For this review, use the dimensioned drawing (mm, ordinates from the lowest corner) and the shaded views. A direction names the side the tool comes from. Coordinates: 2 decimals unless noted, no trailing zeros. Write each loop counter-clockwise with the first axis right and the second up, starting at its lowest first coordinate (ties: lowest second). Pieces come first, ordered by that corner, then holes. Notation, with made-up numbers: (77, 79) -> (125, 79) arc R29 cw to (125, 102) -> close; hole circle Ø7 at (31, -16). An arc over 180 degrees is marked (long way). Put each result on its own line as item: value. Start each with the question number.
Item 1: Consider section D-D on x = 11. Give the boundary of the cut face in (y, z), and give its area (3 significant figures).
Item 2: Consider section A-A on z = 16.5. Give the boundary of the cut face in (x, y).
Item 3: Consider section C-C on x = 3. Give the boundary of the cut face in (y, z), and give its area (3 significant figures).
Item 4: Consider section B-B on y = 2.5. Give the boundary of the cut face in (x, z).
Item 5: For the marked faces 1 and 2, list the 3-axis set-ups (+Z, -Z, +X, -X, +Y, -Y) from which the entire face can be reached by the end or side of a thin tool; tool diameter is ignored.
Item 6: Insertion check: P1, Ø3, axis at x = 21, z = 27.5, coming from the -Y side; P2, Ø9, axis at x = 17.5, z = 25.5, coming from the -Y side; P3, Ø12.5, axis at x = 29, y = 22.5, coming from the +Z side. Each pin has a flat end and moves straight along its axis. Give the tip position at first contact, or say it passes through.
Item 7: To check wall thickness, follow L1, parallel to Y at x = 37, z = 7; L2, parallel to Z at x = 20, y = 30.6; L3, parallel to X at y = 2, z = 3. State the ranges of each line that lie inside material, in increasing order.
Item 8: The part is to be moulded in two halves that separate along Y. For the marked faces 3, 4, 5 and 6, say which applies: +Y half, -Y half, draft (parallel to the pull), parting line (faces both ways), or undercut.
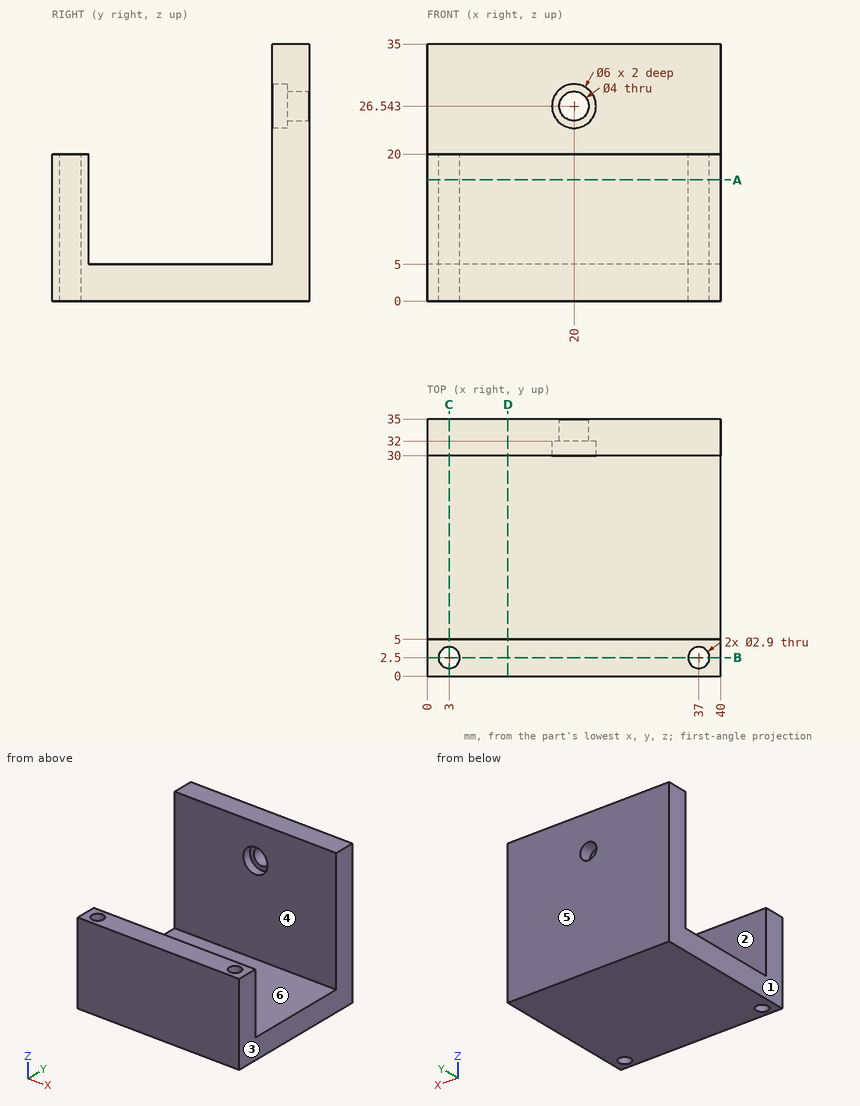
Return value:
1. outline: (0, 0) -> (35, 0) -> (35, 35) -> (30, 35) -> (30, 5) -> (5, 5) -> (5, 20) -> (0, 20) -> close
1. area: 400 mm^2
2. outline: (0, 0) -> (40, 0) -> (40, 5) -> (0, 5) -> close; (0, 30) -> (40, 30) -> (40, 35) -> (0, 35) -> close; hole circle Ø2.9 at (3, 2.5); hole circle Ø2.9 at (37, 2.5)
3. outline: (0, 0) -> (1.05, 0) -> (1.05, 20) -> (0, 20) -> close; (3.95, 0) -> (35, 0) -> (35, 35) -> (30, 35) -> (30, 5) -> (5, 5) -> (5, 20) -> (3.95, 20) -> close
3. area: 342 mm^2
4. outline: (0, 0) -> (1.55, 0) -> (1.55, 20) -> (0, 20) -> close; (4.45, 0) -> (35.55, 0) -> (35.55, 20) -> (4.45, 20) -> close; (38.45, 0) -> (40, 0) -> (40, 20) -> (38.45, 20) -> close
5. face 1: +Z, -Z, -X, +Y, -Y
5. face 2: +Z, +X, -X
6. P1: y = 32
6. P2: y = 30
6. P3: z = 5
7. L1: 0 to 1.05, 3.95 to 5, 30 to 35
7. L2: 0 to 23.54, 29.54 to 35
7. L3: 0 to 1.64, 4.36 to 35.64, 38.36 to 40
8. face 3: draft
8. face 4: undercut
8. face 5: +Y half
8. face 6: undercut
